```python
from build123d import *

# Parameters (mm, degrees)
F0_W     = 127
F0_H     = 127
F1_DEPTH = 50.8
F2_R     = 33.083677
F3_DEPTH = 50.801
F4_R     = 9.812618
F4_R_2   = 12.86692
F4_R_3   = 8.071965
F4_R_4   = 13.073277
F4_R_5   = 22.768833
F5_DEPTH = 12.7


with BuildPart() as f1:
    # F0 (on Top) → F1 (new body)
    with BuildSketch(Plane.XY):
        with Locations((0.94142, -6.859615)):
            Rectangle(F0_W, F0_H)
    extrude(amount=F1_DEPTH)

    # F2 (on face) → F3 (cut, through all)
    with BuildSketch(Plane.XY.offset(50.8)):
        with Locations((0.94142, -6.859615)):
            Circle(F2_R)
    extrude(amount=-F3_DEPTH, mode=Mode.SUBTRACT)

    # F4 (on face) → F5 (cut)
    with BuildSketch(Plane.XY.offset(50.8)):
        with Locations((-51.02095, 41.184627)):
            Circle(F4_R)
        with Locations((45.015216, 42.094678)):
            Circle(F4_R_2)
        with Locations((-41.62769, -50.914697)):
            Circle(F4_R_3)
        with Locations((43.389134, -46.201754)):
            Circle(F4_R_4)
        with Locations((49.104106, 0)):
            Circle(F4_R_5)
    extrude(amount=-F5_DEPTH, mode=Mode.SUBTRACT)


solid = f1.part
```
Input: part model. Units: mm. Frame: model coordinates. A direction names the side the tool comes from. Round coordinates to 2 decimals unless told otherwise and drop trailing zeros. Loops run counter-clockwise (first coordinate to the right, second up) from the corner with the lowest first, then second, coordinate; pieces in that order, holes last. Notation, with made-up numbers: (42, 67.5) - (73, 67.5) arc R23 cw to (73, 85.5) - close; hole circle Ø3 at (-39, 27.5). An arc over 180 degrees is marked (long way). One line per item, written item: value. Start each with the question number.
(1) Section A-A, the plane x = 1.5. Return loops of the section in (y, z).
(2) Ray query, line 1 (X direction, y = -8, z = 12); line 2 (Y direction, x = -37, z = 41); line 3 (Z direction, x = 58, y = -12.5). Return the intervals inside material, ascending. Write a range as [from, to].
(3) Section B-B, the plane y = -3. Return loops of the section in (x, z), plus the area to 3 significant figures.
(4) Draft query along Y for faces 3 (the flat face through (0, 56.64, 25)), 4 (the flat face through (0, -70.36, 25)), 5 (the cylindrical face through (-25.313, -26.991, 25.756)), 6 (the flat face through (28, -34, 0)). Return one class per face: +Y half, -Y half, draft (parallel to the pull), parting line (faces both ways), or undercut.
(5) Section D-D, the plane z = 4. Return loops of the section in (x, y), plus the area to 3 significant figures.
(6) Section C-C, the plane z = 46. Return loops of the section in (x, y), plus the area to 3 significant figures.
(7) Contact query for a flat-ended pin moving along its axis: P1, Ø8, axis at x = 49, y = -47, coming from the +Z side. Output: stop coordinate, or through.
(8) Access query for faces 1 (the flat face through (-28, -34, 50.8)), 2 (the flat face through (43, -46, 38.1)). Directions: +Z, -Z, +X, -X, +Y, -Y. A direction counts if a zero-diameter tool reaches every point of the face in a straight line with its end or side. Return the directions, or none.
Results below:
1. outline: (-70.36, 0) - (-39.94, 0) - (-39.94, 50.8) - (-70.36, 50.8) - close; (26.22, 0) - (56.64, 0) - (56.64, 50.8) - (26.22, 50.8) - close
2. line 1: [-62.56, -32.12], [34.01, 64.44]
2. line 2: [-70.36, -57.53], [-44.3, 56.64]
2. line 3: [0, 38.1]
3. outline: (-62.56, 0) - (-31.92, 0) - (-31.92, 50.8) - (-62.56, 50.8) - close; (33.8, 0) - (64.44, 0) - (64.44, 38.1) - (33.8, 38.1) - close
3. area: 2,720 mm^2
4. face 3: +Y half
4. face 4: -Y half
4. face 5: undercut
4. face 6: draft
5. outline: (-62.56, -70.36) - (64.44, -70.36) - (64.44, 56.64) - (-62.56, 56.64) - close; hole circle Ø66.17 at (0.94, -6.86)
5. area: 12,700 mm^2
6. outline: (-62.56, -70.36) - (64.44, -70.36) - (64.44, -16.83) arc R22.77 cw to (32.78, -15.87) arc R33.08 cw (long way) to (28.99, 10.68) arc R22.77 cw to (64.44, 16.83) - (64.44, 56.64) - (-62.56, 56.64) - close; hole circle Ø19.63 at (-51.02, 41.18); hole circle Ø16.14 at (-41.63, -50.91); hole circle Ø26.15 at (43.39, -46.2); hole circle Ø25.73 at (45.02, 42.09)
6. area: 9,800 mm^2
7. P1: z = 38.1
8. face 1: +Z, +X, -X, +Y, -Y
8. face 2: +Z
